Geometry: final body of the model. Coordinates: model frame, mm. Face numbers are marked on the shaded views. Round coordinates to 2 decimals unless told otherwise and drop trailing zeros. Loops run counter-clockwise (first coordinate to the right, second up) from the corner with the lowest first, then second, coordinate; pieces in that order, holes last. Notation, with made-up numbers: (-10.5, 48) - (44.5, 48) arc R14 ccw to (44.5, 68) - close; hole circle Ø5 at (22.5, 65). An arc over 180 degrees is marked (long way). Answer as CSV lines item,"result".
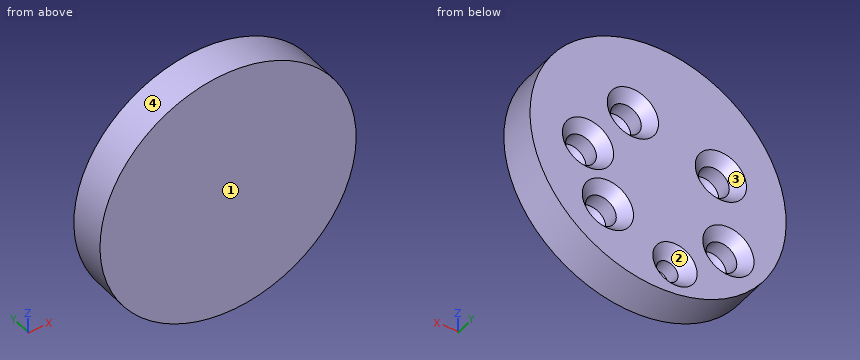
from build123d import *

# Parameters (mm, degrees)
SKETCH1_R                                            = 50
BOSS_EXTRUDE1_DEPTH                                  = 15
CSK_FOR_M10_COUNTERSUNK_FLAT_HEAD_SCREW2_D           = 12
CSK_FOR_M10_COUNTERSUNK_FLAT_HEAD_SCREW2_DEPTH       = 10
CSK_FOR_M10_COUNTERSUNK_FLAT_HEAD_SCREW2_CSINK_D     = 20
CSK_FOR_M10_COUNTERSUNK_FLAT_HEAD_SCREW2_CSINK_ANGLE = 90
CSK_FOR_M10_COUNTERSUNK_FLAT_HEAD_SCREW2_TIP         = 3.605163714
CSK_FOR_M8_COUNTERSUNK_FLAT_HEAD_SCREW1_D            = 8.4
CSK_FOR_M8_COUNTERSUNK_FLAT_HEAD_SCREW1_DEPTH        = 10
CSK_FOR_M8_COUNTERSUNK_FLAT_HEAD_SCREW1_CSINK_D      = 17.3
CSK_FOR_M8_COUNTERSUNK_FLAT_HEAD_SCREW1_CSINK_ANGLE  = 90
CSK_FOR_M8_COUNTERSUNK_FLAT_HEAD_SCREW1_TIP          = 2.5236146


with BuildPart() as part:
    # Sketch1 → Boss-Extrude1 (new body)
    with BuildSketch(Plane(origin=(0, 0, 0), x_dir=(1, 0, 0), z_dir=(0, 1, 0))):
        with Locations(Location((0, 0, 0), (0, 0, 270))):
            Circle(SKETCH1_R)
    extrude(amount=BOSS_EXTRUDE1_DEPTH)

    # CSK for M10 Countersunk Flat Head Screw2
    with Locations(Plane(origin=(0, 15, 0), x_dir=(1, 0, 0), z_dir=(0, 1, 0))):
        with Locations((-27.458630514, 22.136146371), (19.59369175, 24.281141581), (-24.521924649, -7.872760418), (9.832439438, -18.376753366), (27.367685205, 2.373094983)):
            CounterSinkHole(CSK_FOR_M10_COUNTERSUNK_FLAT_HEAD_SCREW2_D / 2, CSK_FOR_M10_COUNTERSUNK_FLAT_HEAD_SCREW2_CSINK_D / 2, depth=CSK_FOR_M10_COUNTERSUNK_FLAT_HEAD_SCREW2_DEPTH, counter_sink_angle=CSK_FOR_M10_COUNTERSUNK_FLAT_HEAD_SCREW2_CSINK_ANGLE)
            with Locations((0, 0, -(CSK_FOR_M10_COUNTERSUNK_FLAT_HEAD_SCREW2_DEPTH + CSK_FOR_M10_COUNTERSUNK_FLAT_HEAD_SCREW2_TIP / 2))):  # 118° drill point
                Cone(0, CSK_FOR_M10_COUNTERSUNK_FLAT_HEAD_SCREW2_D / 2, CSK_FOR_M10_COUNTERSUNK_FLAT_HEAD_SCREW2_TIP, mode=Mode.SUBTRACT)

    # CSK for M8 Countersunk Flat Head Screw1
    with Locations(Plane(origin=(0, 15, 0), x_dir=(1, 0, 0), z_dir=(0, 1, 0))):
        with Locations((-6.596639158, 37.29118486)):
            CounterSinkHole(CSK_FOR_M8_COUNTERSUNK_FLAT_HEAD_SCREW1_D / 2, CSK_FOR_M8_COUNTERSUNK_FLAT_HEAD_SCREW1_CSINK_D / 2, depth=CSK_FOR_M8_COUNTERSUNK_FLAT_HEAD_SCREW1_DEPTH, counter_sink_angle=CSK_FOR_M8_COUNTERSUNK_FLAT_HEAD_SCREW1_CSINK_ANGLE)
            with Locations((0, 0, -(CSK_FOR_M8_COUNTERSUNK_FLAT_HEAD_SCREW1_DEPTH + CSK_FOR_M8_COUNTERSUNK_FLAT_HEAD_SCREW1_TIP / 2))):  # 118° drill point
                Cone(0, CSK_FOR_M8_COUNTERSUNK_FLAT_HEAD_SCREW1_D / 2, CSK_FOR_M8_COUNTERSUNK_FLAT_HEAD_SCREW1_TIP, mode=Mode.SUBTRACT)


solid = part.part
(1) Section B-B (x = -42.5). Output: boundary loops of the cut face in (y, z).
Findings below:
outline,"(0, -26.34) - (15, -26.34) - (15, 26.34) - (0, 26.34) - close"
(2) Pin query (flat end, axial travel): P1, Ø11, axis at x = 27.37, z = -2.37, coming from the +Y side; P2, Ø5, axis at x = 19, y = 8.5, coming from the +Z side; P3, Ø4, axis at x = -6.5, y = 12.5, coming from the +Z side. Return the tip coordinate at first contact, or that it passes through.
Findings below:
P1,"y = 4.7"
P2,"z = 47.2"
P3,"z = 49.8"
(3) Draft query along Z for the marked faces 1, 2, 3 and 4. Return one class per face: pulls with the +Z half, pulls with the -Z half, needs draft (parallel to the pull), parting line crosses it, or undercut.
Findings below:
face 1,"needs draft"
face 2,"undercut"
face 3,"undercut"
face 4,"parting line crosses it"
(4) Section A-A (z = 38.5). Output: boundary loops of the cut face in (x, y), and give its area (3 significant figures).
Findings below:
outline,"(-31.9, 0) - (31.9, 0) - (31.9, 15) - (-31.9, 15) - close"
area,"957 mm2"
(5) Material intervals for line 1 along X through (y, z) = (14, -32); line 2 along Z through (x, y) = (-25.5, 13.75); line 3 along Z through (x, y) = (-29, 12.75), sorted ascending.
Findings below:
line 1,"-38.42 to -12.12, -1.07 to 14.97, 24.22 to 38.42"
line 2,"-43.01 to -30.66, -13.61 to -0.82, 16.57 to 43.01"
line 3,"-40.73 to -29.73, -14.54 to 1.55, 14.2 to 40.73"
